Could you check a few things on this model? Use its own coordinates, in mm. A direction names the side the tool comes from. Give positions to 0.01 mm unless a question says otherwise; leave off trailing zeros. Loops run counter-clockwise (first coordinate to the right, second up) from the corner with the lowest first, then second, coordinate; pieces in that order, holes last.
1. Imagine slicing it at A-A (y = -2.5). List the corners of the cut face in (x, z) for me.
2. I need wall thicknesses on line 1 along X through (y, z) = (-22.5, 29.5); line 2 along Z through (x, y) = (35, -5); line 3 along Z through (x, y) = (36.5, -13.25). Which ranges of each line are inside material? Lowest first, please.
3. For P1, Ø5, axis at y = -18, z = 23, coming from the +X side; P2, Ø8, axis at y = -8.5, z = 30, coming from the +X side, each with a flat end and sliding along its axis, tell me the tip position at first contact or that it passes through.
4. Imagine slicing it at C-C (x = 36). List the corners of the cut face in (y, z) for me, plus the area to 3 significant figures.
5. Imagine slicing it at B-B (z = 33.5). List the corners of the cut face in (x, y) for me, plus the area to 3 significant figures.
6. For faces 1 (the flat face through (0, -13, 26)), 2 (the flat face through (25.4, -13, 38)), which set-ups out of +Z, -Z, +X, -X, +Y, -Y let a thin tool reach every point of the face, with its end or its side?
```python
from build123d import *

# Parameters (mm, degrees)
F1_DEPTH    = 25.4
F2_T1_DEPTH = 195.8114627457


# Not quite as in the source:
# - a fillet or chamfer that OpenCascade refuses, or shapes differently, is made with other operations: its cross-section is extruded or revolved along the edge and cut away or added


with BuildPart() as f1:
    # F0 (on Front) → F1 (new body)
    with BuildSketch(Plane.XZ):
        Polygon((0, 50.8), (0, 0), (50.8, 0), (50.8, 25.4), (25.4, 25.4), (25.4, 50.8), align=None)
    extrude(amount=F1_DEPTH)

    # F2: fillet of radius 35.5661942009 on 1 edges, made by hand

    # F2_s2 → F2_t1 (cut)
    with BuildSketch(Plane.XZ.offset(-85.2057313728)):
        with BuildLine():
            ThreePointArc((50.8, -8.6822925491), (43.7515810206, 12.5707229158), (25.4, 25.4))
            Line((25.4, 25.4), (25.603323884, 26.081645851))
            ThreePointArc((25.603323884, 26.081645851), (38.1, 26.111323884), (50.8, 26.111323884))
            Line((50.8, 26.111323884), (51.511323884, 25.4))
            Line((51.511323884, 25.4), (51.511323884, -8.6822925491))
            Line((51.511323884, -8.6822925491), (50.8, -8.6822925491))
        make_face()
    extrude(amount=F2_T1_DEPTH, mode=Mode.SUBTRACT)


solid = f1.part
```
Derived:
1. outline: (0, 0) - (49.72, 0) arc R35.57 ccw to (25.4, 25.4) - (25.4, 50.8) - (0, 50.8) - close
2. line 1: x = 0 to 25.4
2. line 2: z = 0 to 20.89
2. line 3: z = 0 to 19.83
3. P1: stops at x = 35.56
3. P2: stops at x = 25.4
4. outline: (-25.4, 0) - (0, 0) - (0, 20.19) - (-25.4, 20.19) - close
4. area: 513 mm2
5. outline: (0, -25.4) - (25.4, -25.4) - (25.4, 0) - (0, 0) - close
5. area: 645 mm2
6. face 1: +Z, -Z, -X, +Y, -Y
6. face 2: +Z, +X, +Y, -Y
